```python
from build123d import *

# Parameters (mm, degrees)
SKETCH_1_R                = 16
EXTRUDE_1_DEPTH           = 5
F_3_0MM_1_D               = 3
F_3_0MM_1_DEPTH           = 3
F_3_0MM_1_TIP             = 0.901290929
HOLE_WIZARD_1_D           = 3.2
HOLE_WIZARD_1_DEPTH       = 5
HOLE_WIZARD_1_CBORE_D     = 5.8
HOLE_WIZARD_1_CBORE_DEPTH = 3
HOLE_WIZARD_1_TIP         = 0.96137699
EXTRUDE_2_DEPTH           = 5
SKETCH_9_W                = 3
SKETCH_9_H                = 46
EXTRUDE_3_DEPTH           = 46.5
SKETCH_12_R               = 1.6
CUT_EXTRUDE_1_DEPTH       = 45
CUT_EXTRUDE_2_DEPTH       = 62.483737687
SKETCH_17_W               = 28.420595315
SKETCH_17_H               = 5
CUT_EXTRUDE_3_DEPTH       = 59.908827861
FILLET_3_R                = 6
FILLET_4_R                = 3
FILLET_5_R                = 1
FILLET_6_R                = 8
CUT_EXTRUDE_4_DEPTH       = 64.326534875
CUT_EXTRUDE_4_DEPTH_BACK  = 64.326534875
SKETCH_18_W               = 60.691939919
SKETCH_18_H               = 58.869698126
SKETCH_19_R               = 7.5
CUT_EXTRUDE_5_DEPTH       = 55.591666189
CHAMFER_1_SIZE            = 0.5


with BuildPart() as part:
    # 草图1 → 凸台-拉伸1 (new body)
    with BuildSketch(Plane.XY):
        Circle(SKETCH_1_R)
    extrude(amount=EXTRUDE_1_DEPTH)

    # Ø3.0mm 暗销孔1
    with Locations(Plane.XY.offset(5)):
        with Locations((0, 12), (10.392304845, -6), (-10.392304845, -6)):
            Hole(F_3_0MM_1_D / 2, depth=F_3_0MM_1_DEPTH)
            with Locations((0, 0, -(F_3_0MM_1_DEPTH + F_3_0MM_1_TIP / 2))):  # 118° drill point
                Cone(0, F_3_0MM_1_D / 2, F_3_0MM_1_TIP, mode=Mode.SUBTRACT)

    # 孔1
    with Locations(Plane(origin=(0, 0, 0), x_dir=(-1, 0, 0), z_dir=(0, 0, -1))):
        with Locations((0, -12), (-10.392304845, 6), (10.392304845, 6)):
            CounterBoreHole(HOLE_WIZARD_1_D / 2, HOLE_WIZARD_1_CBORE_D / 2, HOLE_WIZARD_1_CBORE_DEPTH, depth=HOLE_WIZARD_1_DEPTH)
            with Locations((0, 0, -(HOLE_WIZARD_1_DEPTH + HOLE_WIZARD_1_TIP / 2))):  # 118° drill point
                Cone(0, HOLE_WIZARD_1_D / 2, HOLE_WIZARD_1_TIP, mode=Mode.SUBTRACT)

    # 草图8 → 凸台-拉伸2 (add)
    with BuildSketch(Plane.XY):
        with BuildLine():
            Line((0, 23), (17, 23))
            Line((17, 23), (17, -23))
            Line((17, -23), (0, -23))
            Line((0, -23), (0, -16))
            ThreePointArc((0, -16), (16, 0), (0, 16))
            Line((0, 16), (0, 23))
        make_face()
    extrude(amount=EXTRUDE_2_DEPTH)

    # 草图9 → 凸台-拉伸3 (add)
    with BuildSketch(Plane(origin=(0, 0, 0), x_dir=(-1, 0, 0), z_dir=(0, 0, -1))):
        with Locations((-15.5, 0)):
            Rectangle(SKETCH_9_W, SKETCH_9_H)
    extrude(amount=EXTRUDE_3_DEPTH)

    # 草图12 → 切除-拉伸1 (cut)
    with BuildSketch(Plane(origin=(17, 0, 0), x_dir=(0, 0, -1), z_dir=(1, 0, 0))):
        with Locations(Location((3.285846384, 13.959899742, 0), (0, 0, 90))):
            Circle(SKETCH_12_R)
        with Locations(Location((36.459899742, 19.214153616, 0), (0, 0, 90))):
            Circle(SKETCH_12_R)
        with Locations(Location((41.714153616, -13.959899742, 0), (0, 0, 90))):
            Circle(SKETCH_12_R)
        with Locations(Location((8.540100258, -19.214153616, 0), (0, 0, 90))):
            Circle(SKETCH_12_R)
    extrude(amount=-CUT_EXTRUDE_1_DEPTH, mode=Mode.SUBTRACT)

    # 草图14 → 切除-拉伸2 (cut, through all)
    with BuildSketch(Plane(origin=(17, 0, 0), x_dir=(0, 0, -1), z_dir=(1, 0, 0))):
        with BuildLine():
            Line((7.285846384, 23), (7.285846384, 16.255659243))
            ThreePointArc((7.285846384, 16.255659243), (6.878739032, 13.431405246), (5.690564256, 10.837106162))
            ThreePointArc((5.690564256, 10.837106162), (10.391665009, -15.918172751), (37.430987945, -13.306599828))
            ThreePointArc((37.430987945, -13.306599828), (40.805821772, -10.83485182), (44.896481918, -9.959899742))
            Line((44.896481918, -9.959899742), (46.5, -9.959899742))
            Line((46.5, -9.959899742), (46.5, 23))
            Line((46.5, 23), (7.285846384, 23))
        make_face()
    extrude(amount=-CUT_EXTRUDE_2_DEPTH, mode=Mode.SUBTRACT)

    # 草图17 → 切除-拉伸3 (cut, through all)
    with BuildSketch(Plane.XY.offset(5)):
        with Locations((14.210297658, 20.5)):
            Rectangle(SKETCH_17_W, SKETCH_17_H)
    extrude(amount=-CUT_EXTRUDE_3_DEPTH, mode=Mode.SUBTRACT)

    # 圆角3
    # the kernel refuses this fillet: 6 mm, written as the material it adds along each edge
    with BuildSketch(Plane(origin=(0, -16, 0), x_dir=(-0.9904775075289876, 0.1376746421065417, 0), z_dir=(0, 0, 1))) as fillet_3_piece_1:
        with BuildLine():
            CenterArc((5.2316364, 5.942865045), FILLET_3_R, 187.913310066, 74.173379868)
            Line((-0.711228645, 5.116817193), (-0.830085946, 5.100296235))
            Line((-0.830085946, 5.100296235), (-0.118857301, -0.016520957))
            Line((-0.118857301, -0.016520957), (0.016520957, -0.118857301))
            ThreePointArc((0.016520957, -0.118857301), (2.202794274, 0.03235988), (4.38906759, -0.118857301))
            Line((4.38906759, -0.118857301), (4.405588547, 0))
        make_face()
    extrude(amount=5)
    with BuildSketch(Plane(origin=(0, 16, 0), x_dir=(-0.993666814064824, -0.11236664374387297, 0), z_dir=(0, 0, 1))) as fillet_3_piece_2:
        with BuildLine():
            CenterArc((4.269932462, -5.962000884), FILLET_3_R, 96.45176027, 42.061664666)
            Line((-0.224733287, -1.987333628), (-0.314626602, -1.907840283))
            ThreePointArc((-0.314626602, -1.907840283), (-0.231606661, -0.980182817), (-0.119240018, 0.013483997))
            Line((-0.119240018, 0.013483997), (0.013483997, 0.119240018))
            ThreePointArc((0.013483997, 0.119240018), (1.7978663, 0.018669025), (3.582248603, 0.119240018))
            Line((3.582248603, 0.119240018), (3.5957326, 0))
        make_face()
    extrude(amount=5)
    # the kernel refuses this fillet: 6 mm, written as the material it takes off along each edge
    with BuildSketch(Plane(origin=(27.207517679, -9.959899742, -46.5), x_dir=(0, 0, 1), z_dir=(-1, 0, 0))) as fillet_3_2_piece_1:
        with BuildLine():
            CenterArc((6, -4.083007072), FILLET_3_R, 137.117180669, 42.882819331)
            Line((0, -4.083007072), (-0.12, -4.083007072))
            Line((-0.12, -4.083007072), (-0.12, 0))
            Line((-0.12, 0), (0, 0.12))
            ThreePointArc((0, 0.12), (0.801759041, 0.12), (1.515588444, 0.081660141))
            Line((1.515588444, 0.081660141), (1.603518082, 0))
        make_face()
    extrude(amount=23.415035358, mode=Mode.SUBTRACT)
    with BuildSketch(Plane(origin=(3.426044847, 18, -7.285846384), x_dir=(0, 0, 1), z_dir=(1, 0, 0))) as fillet_3_2_piece_2:
        with BuildLine():
            CenterArc((4.229582061, 6), FILLET_3_R, 225.176083116, 44.823916884)
            Line((0, 1.744340757), (-0.084591641, 1.659227573))
            ThreePointArc((-0.084591641, 1.659227573), (-0.12, 0.872170379), (-0.12, 0))
            Line((-0.12, 0), (0, -0.12))
            Line((0, -0.12), (4.229582061, -0.12))
            Line((4.229582061, -0.12), (4.229582061, 0))
        make_face()
    extrude(amount=24.147910306, mode=Mode.SUBTRACT)

    # 圆角4
    fillet_4_edges = [part.edges().sort_by_distance(p)[0] for p in [
        (17, -2.5, 5),
        (15.5, -9.959899742, -44.896481918),
        (0, -23, 2.5),
        (0, 18, 2.5),
        (15.5, 16.255659243, -7.285846384),
    ]]
    fillet(fillet_4_edges, radius=FILLET_4_R)

    # 圆角5
    fillet_5_edges = [part.edges().sort_by_distance(p)[0] for p in [
        (14, -2.5, 0),
    ]]
    fillet(fillet_5_edges, radius=FILLET_5_R)

    # 圆角6
    fillet_6_edges = [part.edges().sort_by_distance(p)[0] for p in [
        (15.5, -23, -46.5),
    ]]
    fillet(fillet_6_edges, radius=FILLET_6_R)


with BuildPart() as body_2:
    # 镜向1: mirrored copy
    add(part.part.mirror(Plane.XY.offset(5)))

    # 草图19 → 切除-拉伸5 (cut, through all)
    with BuildSketch(Plane.XY.offset(10)):
        Circle(SKETCH_19_R)
    extrude(amount=-CUT_EXTRUDE_5_DEPTH, mode=Mode.SUBTRACT)

    # 倒角1
    chamfer_1_edges = [body_2.edges().sort_by_distance(p)[0] for p in [
        (17, -15.918172751, 20.391665009),
        (17, -11.343083088, 49.821989751),
        (17, 18, 10.528132161),
        (17, -14.521453407, 56.5),
        (17, -13.120063884, 56.42860531),
        (14, 17.899238657, 14.151245267),
        (-15.994794668, 0.408097436, 5),
        (-15.994794668, 0.408097436, 10),
        (-1.458623572, -17.244798923, 5),
        (-2.041852688, 16.175901434, 10),
        (8.462074056, -23, 5),
        (7.962074056, -23, 10),
        (17, -23, 28.25),
        (16.121320344, -23, 5.878679656),
        (7.184813213, 18, 10),
        (-1.458623572, -17.244798923, 10),
        (0.239238095, 17.778888667, 10),
        (0.94500821, -22.254552116, 10),
        (7.684813213, 18, 5),
        (-2.041852688, 16.175901434, 5),
        (0.239238095, 17.778888667, 5),
        (0.94500821, -22.254552116, 5),
        (16.121320344, 18, 5.878679656),
        (17, 12.444073597, 16.530943185),
        (14, 12.444073597, 16.530943185),
        (17, 17.899238657, 14.151245267),
        (17, -10.527865197, 54.849185717),
        (17, 16.230924248, 16.769699588),
        (14, -13.120063884, 56.42860531),
        (14, -10.527865197, 54.849185717),
        (14, 16.230924248, 16.769699588),
        (14, 18, 12.028132161),
        (13.707106781, 18, 10.292893219),
        (13.707106781, -23, 10.292893219),
        (14, -14.521453407, 56.5),
        (14, -23, 29.75),
        (14, -20.656854249, 54.156854249),
        (17, -20.656854249, 54.156854249),
        (-7.5, 0, 5),
        (-7.5, 0, 10),
        (14, -15.918172751, 20.391665009),
        (14, -11.343083088, 49.821989751),
    ]]
    chamfer(chamfer_1_edges, length=CHAMFER_1_SIZE)


with BuildPart() as part_1:
    add(part.part)

    # 草图18 → 切除-拉伸4 (cut, two sides: drawn at the far end of the back side and taken through both)
    with BuildSketch(Plane(origin=(0, 0, 0), x_dir=(1, 0, 0), z_dir=(0, 1, 0)).offset(-CUT_EXTRUDE_4_DEPTH_BACK)):
        with Locations((-2.212398845, 24.434849063)):
            Rectangle(SKETCH_18_W, SKETCH_18_H)
    extrude(amount=CUT_EXTRUDE_4_DEPTH + CUT_EXTRUDE_4_DEPTH_BACK, mode=Mode.SUBTRACT)


solid = body_2.part
```
Input: part model. Units: mm. Frame: model coordinates. A direction names the side the tool comes from. Coordinates: 2 decimals unless noted, no trailing zeros. Use a Markdown table: item, result.
1) Pull-direction query (Y, two-part tool) for faces 1 (the cylindrical face through (-2.062, 16.165, 7.528)), 2 (the cylindrical face through (11.89, -5.93, 6.52)), 3 (the conical face through (14.14, -20.34, 53.96)); classes: released by +Y, released by -Y, zero draft, split by the parting line, or undercut.
Results found:
| item | result |
|---|---|
| face 1 | released by +Y |
| face 2 | undercut |
| face 3 | released by -Y |
2) Contact query for flat-ended pins moving along their axis: pin 1 (7.5 mm diameter, centred on x = 0, y = -12, fed in from +Z); pin 2 (4 mm diameter, centred on y = -19.21, z = 18.54, fed in from -X); pin 3 (5 mm diameter, centred on x = -10.39, y = 6, fed in from +Z). Output: stop coordinate, or through.
Results found:
| item | result |
|---|---|
| pin 1 | stops at z = 10 |
| pin 2 | stops at x = 14 |
| pin 3 | stops at z = 7 |
3) Access query for faces 4 (the conical face through (-10.599, -6.159, 8.745)), 5 (the cylindrical face through (13.29, 6.13, 8.52)). Directions: +Z, -Z, +X, -X, +Y, -Y. A direction counts if a zero-diameter tool reaches every point of the face in a straight line with its end or side. Return the directions, or none.
Results found:
| item | result |
|---|---|
| face 4 | -Z |
| face 5 | +Z |
4) Material intervals for line 1 along X through (y, z) = (6, 6.3); line 2 along Z through (x, y) = (6, 6); line 3 along Z through (x, y) = (1.5, -14), sorted ascending. Write a range as from..to.
Results found:
| item | result |
|---|---|
| line 1 | x = -14.83..-11.99, -8.79..-4.5, 4.5..8.79, 11.99..16.47 |
| line 2 | z = 5..10 |
| line 3 | z = 5..7 |
5) Cut plane A-A (y = 6). Give the number of separate pieces and of enclosed holes in the cut face, then the cut area to 3 significant figures.
Results found:
| item | result |
|---|---|
| separate pieces | 4 |
| enclosed holes | 0 |
| area | 73.7 mm2 |
